from build123d import *

# Parameters (mm, degrees)
ESQUISSE1_W                    = 27
ESQUISSE1_H                    = 26
ESQUISSE1_W_2                  = 10
ESQUISSE1_H_2                  = 10
BOSS_EXTRU_1_DEPTH             = 1
ESQUISSE2_W                    = 27
ESQUISSE2_H                    = 26
ESQUISSE2_W_2                  = 25.4
ESQUISSE2_H_2                  = 24.4
BOSS_EXTRU_2_DEPTH             = 5.5
ENL_V_MAT_EXTRU_1_REACH        = 32.008
ESQUISSE3_W                    = 21
ESQUISSE3_H                    = 4
ESQUISSE4_R                    = 1.6
BOSS_EXTRU_3_DEPTH             = 2
R_P_TITION_LIN_AIRE1_COUNT     = 2
R_P_TITION_LIN_AIRE1_PITCH     = 8
R_P_TITION_LIN_AIRE1_COL_COUNT = 2
R_P_TITION_LIN_AIRE1_COL_PITCH = 8


with BuildPart() as part:
    # Esquisse1 → Boss.-Extru.1 (new body)
    with BuildSketch(Plane.XY):
        with Locations((0, 13)):
            Rectangle(ESQUISSE1_W, ESQUISSE1_H)
        with Locations((0, 11)):
            Rectangle(ESQUISSE1_W_2, ESQUISSE1_H_2, mode=Mode.SUBTRACT)
    extrude(amount=BOSS_EXTRU_1_DEPTH)

    # Esquisse2 → Boss.-Extru.2 (add)
    with BuildSketch(Plane.XY.offset(1)):
        with Locations((0, 13)):
            Rectangle(ESQUISSE2_W, ESQUISSE2_H)
        with Locations((0, 13)):
            Rectangle(ESQUISSE2_W_2, ESQUISSE2_H_2, mode=Mode.SUBTRACT)
    extrude(amount=BOSS_EXTRU_2_DEPTH)

    # Esquisse3 → Enlèv. mat.-Extru.1 (cut, up to next)
    with BuildSketch(Plane.XZ, mode=Mode.PRIVATE) as enl_v_mat_extru_1_sk1:
        with Locations((0, 4.5)):
            Rectangle(ESQUISSE3_W, ESQUISSE3_H)
    enl_v_mat_extru_1_tool1 = extrude(enl_v_mat_extru_1_sk1.sketch, amount=-ENL_V_MAT_EXTRU_1_REACH, mode=Mode.PRIVATE) & part.part
    add(enl_v_mat_extru_1_tool1.solids().sort_by_distance((0, 0, 4.5))[0], mode=Mode.SUBTRACT)

    # Esquisse4 → Boss.-Extru.3 (add, symmetric)
    with BuildSketch(Plane(origin=(0, 0, 0), x_dir=(0, 0, -1), z_dir=(1, 0, 0))):
        with BuildLine():
            Line((0, -8), (0, -10.958039892))
            ThreePointArc((0, -10.958039892), (-5.291287847, -12.894531565), (-2.5, -8))
            Line((-2.5, -8), (-2.5, 0))
            Line((-2.5, 0), (0, 0))
            Line((0, 0), (0, -8))
        make_face()
        with Locations((-3, -10.958039892)):
            Circle(ESQUISSE4_R, mode=Mode.SUBTRACT)
    boss_extru_3 = extrude(amount=BOSS_EXTRU_3_DEPTH, both=True)

    # Répétition linéaire1: Boss.-Extru.3 ×2
    with Locations(*[(-i * R_P_TITION_LIN_AIRE1_PITCH, 0, 0) for i in range(1, R_P_TITION_LIN_AIRE1_COUNT)]):
        add(boss_extru_3)

    # Répétition linéaire1 col: Boss.-Extru.3 ×2
    with Locations(*[(i * R_P_TITION_LIN_AIRE1_COL_PITCH, 0, 0) for i in range(1, R_P_TITION_LIN_AIRE1_COL_COUNT)]):
        add(boss_extru_3)


solid = part.part
CAD build for the part. Positions are in the model's coordinates, mm. A direction names the side the tool comes from. Round coordinates to 2 decimals unless told otherwise and drop trailing zeros. Write each loop counter-clockwise with the first axis right and the second up, starting at its lowest first coordinate (ties: lowest second). Pieces come first, ordered by that corner, then holes.
(1) Slice it at D-D, the plane x = 1.25. Write the cut outline in (y, z), and give its area (3 significant figures).
(2) Probe line 1 along Y through (x, z) = (7.05, 3); line 2 along X through (y, z) = (-4.5, 0.5); line 3 along Y through (x, z) = (11.5, 4.25). List the from-to ranges inside material, lowest first.
(3) Slice it at B-B, the plane y = -6. Write the cut outline in (x, z).
(4) Mould opens along Z. For faces 6 (the face through (-8.03, -9.37, 3.21)), 7 (the face through (7.97, -9.37, 3.21)), 8 (the face through (-6, 12, 0)), 9 (the face through (0, 26, 3)) say: pulls with the +Z half, pulls with the -Z half, needs draft (parallel to the pull), parting line crosses it, or undercut.
(5) Drop flat-ended pins along their axis: P1, Ø3, axis at x = -5, z = 1, coming from the -Y side; P2, Ø4, axis at x = -8.5, y = 6, coming from the -Z side; P3, Ø1, axis at x = -4, z = 1.5, coming from the -Y side; P4, Ø3, axis at x = 8.5, y = 14, coming from the +Z side. Give the stop position or say it passes through.
(6) Slice it at A-A, the plane x = -9. Write the cut outline in (y, z), and give its area (3 significant figures).
(7) 3-axis set-ups, long thin cutter, end or side, ignore diameter. For faces 1 (the face through (10.5, 0.4, 4.5)), 2 (the face through (-12.7, 13, 4)), 3 (the face through (-6, -7, 2)), 4 (the face through (-0.1, 6, 0.5)), 5 (the face through (10, -7, 2)): which of +Z, -Z, +X, -X, +Y, -Y reach the whole face in a straight line?
(8) Slice it at C-C, the plane x = -4. Write the cut outline in (y, z).
From the geometry:
1. outline: (-10.96, 0) - (6, 0) - (6, 1) - (0.8, 1) - (0.8, 2.5) - (-8, 2.5) arc R3 ccw (long way) to start; (16, 0) - (26, 0) - (26, 6.5) - (25.2, 6.5) - (25.2, 1) - (16, 1) - close; hole circle Ø3.2 at (-10.96, 3)
1. area: 63.7 mm2
2. line 1: y = -13.96 to -12.56, -9.36 to -7.96, 25.2 to 26
2. line 2: x = -10 to -6, -2 to 2, 6 to 10
2. line 3: y = 0 to 0.8, 25.2 to 26
3. outline: (-10, 0) - (-6, 0) - (-6, 2.5) - (-10, 2.5) - close; (-2, 0) - (2, 0) - (2, 2.5) - (-2, 2.5) - close; (6, 0) - (10, 0) - (10, 2.5) - (6, 2.5) - close
4. face 6: undercut
4. face 7: undercut
4. face 8: pulls with the -Z half
4. face 9: needs draft
5. P1: stops at y = -13.83
5. P2: stops at z = 0
5. P3: stops at y = 0
5. P4: stops at z = 1
6. outline: (-10.96, 0) - (26, 0) - (26, 6.5) - (25.2, 6.5) - (25.2, 1) - (0.8, 1) - (0.8, 2.5) - (-8, 2.5) arc R3 ccw (long way) to start; hole circle Ø3.2 at (-10.96, 3)
6. area: 73.7 mm2
7. face 1: +Z, -Y
7. face 2: +Z
7. face 3: +Z, -Z, -Y
7. face 4: +Z, -Z
7. face 5: +Z, -Z, +X, -Y
8. outline: (0, 0) - (6, 0) - (6, 1) - (0.8, 1) - (0.8, 2.5) - (0, 2.5) - close; (16, 0) - (26, 0) - (26, 6.5) - (25.2, 6.5) - (25.2, 1) - (16, 1) - close
